from build123d import *

# Parameters (mm, degrees)
SKETCH1_W           = 127
SKETCH1_H           = 127
BOSS_EXTRUDE1_DEPTH = 6.35
SKETCH2_R           = 57.15
BOSS_EXTRUDE2_DEPTH = 209.55
SKETCH3_R           = 26.67
BOSS_EXTRUDE3_DEPTH = 33.02


with BuildPart() as part:
    # Sketch1 → Boss-Extrude1 (new body)
    with BuildSketch(Plane.XY):
        Rectangle(SKETCH1_W, SKETCH1_H)
    extrude(amount=BOSS_EXTRUDE1_DEPTH)

    # Sketch2 → Boss-Extrude2 (add)
    with BuildSketch(Plane.XY.offset(6.35)):
        Circle(SKETCH2_R)
    extrude(amount=BOSS_EXTRUDE2_DEPTH)

    # Sketch3 → Boss-Extrude3 (add)
    with BuildSketch(Plane.XY.offset(215.9)):
        Circle(SKETCH3_R)
    extrude(amount=BOSS_EXTRUDE3_DEPTH)


solid = part.part
The listing builds one solid part. Answer for the finished solid, in the listing's coordinates (mm). A direction names the side the tool comes from. Coordinates: 2 decimals unless noted, no trailing zeros. Write each loop counter-clockwise with the first axis right and the second up, starting at its lowest first coordinate (ties: lowest second). Pieces come first, ordered by that corner, then holes. Notation, with made-up numbers: (20, 61.25) - (57, 61.25) arc R26 cw to (57, 81.25) - close; hole circle Ø10 at (-18, 2.5). An arc over 180 degrees is marked (long way). Answer as CSV lines item,"result".
1. Straight lines are drawn through the part: line 1 (Z direction, x = -34.5, y = 16.5); line 2 (Y direction, x = 2, z = 12) (3 decimals); line 3 (Z direction, x = -47, y = -41.5). For each, find the intervals that lie inside material, in ascending order. Write a range as [from, to].
Computed values:
line 1,"z = [0, 215.9]"
line 2,"y = [-57.115, 57.115]"
line 3,"z = [0, 6.35]"
2. Find section A-A (x = 0). Give the vertices of the cut face in (y, z), plus the area to 3 significant figures.
Computed values:
outline,"(-63.5, 0) - (63.5, 0) - (63.5, 6.35) - (57.15, 6.35) - (57.15, 215.9) - (26.67, 215.9) - (26.67, 248.92) - (-26.67, 248.92) - (-26.67, 215.9) - (-57.15, 215.9) - (-57.15, 6.35) - (-63.5, 6.35) - close"
area,"26,500 mm²"
3. Find section B-B (y = -18). Give the vertices of the cut face in (x, z), plus the area to 3 significant figures.
Computed values:
outline,"(-63.5, 0) - (63.5, 0) - (63.5, 6.35) - (54.24, 6.35) - (54.24, 215.9) - (19.68, 215.9) - (19.68, 248.92) - (-19.68, 248.92) - (-19.68, 215.9) - (-54.24, 215.9) - (-54.24, 6.35) - (-63.5, 6.35) - close"
area,"24,800 mm²"
4. Find section D-D (x = 39). Give the vertices of the cut face in (y, z), plus the area to 3 significant figures.
Computed values:
outline,"(-63.5, 0) - (63.5, 0) - (63.5, 6.35) - (41.77, 6.35) - (41.77, 215.9) - (-41.77, 215.9) - (-41.77, 6.35) - (-63.5, 6.35) - close"
area,"18,300 mm²"
5. Find section C-C (z = 30). Give the vertices of the cut face in (x, y).
Computed values:
outline,"circle Ø114.3 at (0, 0)"
6. A tool of negligible diameter and unlimited length cuts with its end or side. For faces 1 (the flat face through (-1, 63.5, 3)), 2 (the cylindrical face through (-57.095, 2.513, 109.658)), from which of +Z, -Z, +X, -X, +Y, -Y can it reach the whole face along a straight path? Write none if from no direction.
Computed values:
face 1,"+Z, -Z, +X, -X, +Y"
face 2,"+Z"
7. Given P1, Ø4, axis at x = -51, y = 32.5, coming from the +Z side; P2, Ø2, axis at x = 40, z = 28.5, coming from the +Y side; P3, Ø4, axis at x = -2, z = 169, coming from the +Y side; P4, Ø10, axis at x = -46.5, y = 2.5, coming from the -Z side, each flat-ended and moving along its own axis, determine where each tip first touches the part or whether it passes through.
Computed values:
P1,"stops at z = 6.35"
P2,"stops at y = 41.77"
P3,"stops at y = 57.15"
P4,"stops at z = 0"
